Work out the finished part from the listing and answer in its coordinate system (mm). A direction names the side the tool comes from. Round coordinates to 2 decimals unless told otherwise and drop trailing zeros. Order: outer loops, then holes, each group sorted by start corner. A loop starts at its lowest first (then second) coordinate and runs counter-clockwise, first axis right, second up. Notation, with made-up numbers: (42.5, -9.75) - (75.5, -9.75) arc R17 ccw to (75.5, 22.25) - close; hole circle Ø7 at (3, -39). An arc over 180 degrees is marked (long way). Answer in a Markdown table with one row per item.
Autodesk Inventor part; units mm, degrees
ref_plane "YZ Plane" through (0, 0, 0) normal (1, 0, 0) x (0, 1, 0)
ref_plane "XZ Plane" through (0, 0, 0) normal (0, 1, 0) x (-1, 0, 0)
ref_plane "XY Plane" through (0, 0, 0) normal (0, 0, 1) x (1, 0, 0)
sketch "Sketch1" plane through (0, 0, 0) normal (0, 1, 0) x (-1, 0, 0)
  line L0 (0, 0) -> (-34, 0)
  line L1 (-34, 0) -> (-34, 34)
  line L2 (-34, 34) -> (0, 34)
  line L3 (0, 34) -> (0, 0)
  dimension "d0" = 34
  dimension "d1" = 34
extrude "Extrusion1" add sketch "Sketch1" along normal blind 33
sketch "Sketch2" plane through (0, 33, 0) normal (0, 1, 0) x (1, 0, 0)
  line L0 (0, -34) -> (34, -34)
  line L1 (34, -34) -> (34, 0)
  line L2 (34, 0) -> (0, 0)
  line L3 (0, 0) -> (0, -34)
  line L4 (2, -2) -> (32, -2)
  line L5 (32, -2) -> (32, -32)
  line L6 (32, -32) -> (2, -32)
  line L7 (2, -32) -> (2, -2)
  dimension "d4" = 2
extrude "Extrusion2" cut sketch "Sketch2" against normal blind 36 contours L4 L5 L6 L7
sketch "Sketch3" plane through (34, 0, 34) normal (1, 0, 0) x (0, 0, -1)
  line L0 (0, 0) -> (34, 0)
  line L1 (0, 33) -> (34, 33)
  line L2 (2, 33) -> (32, 33)
  line L3 (34, 0) -> (34, 38)
  line L4 (34, 0) -> (29, 0)
  line L5 (0, 0) -> (34, 0)
  line L6 (29, 0) -> (29, 4)
  line L7 (34, 0) -> (34, 33)
  line L8 (0, 0) -> (0, 33)
  line L9 (32, 0) -> (2, 0)
  line L10 (32, 33) -> (32, 0)
  line L11 (2, 33) -> (2, 0)
  dimension "d7" = 5
  dimension "d8" = 4
hole "Hole1" at (34, 4, 5) direction (-1, 0, 0) diameter 4 depth 2
ref_plane "Work Plane1" through (17, 33, 32) normal (1, 0, 0) x (0, 0, -1)
mirror "Mirror1" about plane through (17, 33, 32) normal (1, 0, 0) of "Hole1"
sketch "Sketch6" plane through (0, 33, 0) normal (0, 1, 0) x (1, 0, 0)
  point P0 (0, 0)
sketch "Sketch7" plane through (0, 0, 0) normal (0, -1, 0) x (1, 0, 0)
  line L0 (34, 0) -> (0, 0)
  line L1 (0, 34) -> (34, 34)
  line L2 (34, 0) -> (0, 0)
  line L3 (0, 0) -> (0, 34)
  line L4 (0, 34) -> (34, 34)
  line L5 (34, 34) -> (34, 0)
extrude "Extrusion5" add sketch "Sketch7" against normal blind 2
equation "\"BendRadius\" = Thickness"
equation "\"BendReliefWidth\" = Thickness"
equation "\"BendReliefDepth\" = 0.5 * Thickness"
equation "\"CornerReliefSize\" = 4 * Thickness"
equation "\"MinimumRemnant\" = 2 * Thickness"
equation "\"TransitionRadius\" = BendRadius"
equation "\"JacobiRadiusSize\" = Thickness"
equation "\"GapSize\" = Thickness"
properties part number "waterBallonHolderv1"
1) Find section D-D, the plane z = 13. Give the vertices of the cut face in (x, y), then the cut area to 3 significant figures.
Filled in:
| item | result |
|---|---|
| outline | (0, 0) - (34, 0) - (34, 33) - (32, 33) - (32, 2) - (2, 2) - (2, 33) - (0, 33) - close |
| area | 192 mm^2 |
2) The mould has two halves that part along Z. Classify faces 3 (the face through (1, 2, 5)), 4 (the face through (17, 16, 0)), 5 (the face through (34, 16, 17)), 6 (the face through (17, 2, 17)): released by +Z, released by -Z, zero draft, split by the parting line, or undercut.
Filled in:
| item | result |
|---|---|
| face 3 | undercut |
| face 4 | released by -Z |
| face 5 | zero draft |
| face 6 | undercut |
3) Find section B-B, the plane x = 26. Give the vertices of the cut face in (y, z).
Filled in:
| item | result |
|---|---|
| outline | (0, 0) - (33, 0) - (33, 2) - (2, 2) - (2, 32) - (33, 32) - (33, 34) - (0, 34) - close |
4) Each of these flat-tipped pins is pushed along its axis until it touches: pin 1 (8 mm diameter, centred on x = 7, z = 16, fed in from +Y); pin 2 (3 mm diameter, centred on y = 4, z = 5, fed in from -X). Where does it stop, or does it pass through?
Filled in:
| item | result |
|---|---|
| pin 1 | stops at y = 2 |
| pin 2 | passes through |
5) Find the intervals of material crossed by probe 1 along X at (y, z) = (20.5, 19); probe 2 along Y at (x, z) = (32.6, 5); probe 3 along Z at (x, y) = (1.45, 4), in increasing order. Write a range as from..to.
Filled in:
| item | result |
|---|---|
| probe 1 | x = 0..2, 32..34 |
| probe 2 | y = 0..2, 6..33 |
| probe 3 | z = 0..3, 7..34 |
6) Find section C-C, the plane y = 4. Give the vertices of the cut face in (x, z), then the cut area to 3 significant figures.
Filled in:
| item | result |
|---|---|
| outline | (0, 0) - (34, 0) - (34, 3) - (32, 3) - (32, 2) - (2, 2) - (2, 3) - (0, 3) - close; (0, 7) - (2, 7) - (2, 32) - (32, 32) - (32, 7) - (34, 7) - (34, 34) - (0, 34) - close |
| area | 240 mm^2 |
7) Find section A-A, the plane y = 27.5. Give the vertices of the cut face in (x, z).
Filled in:
| item | result |
|---|---|
| outline | (0, 0) - (34, 0) - (34, 34) - (0, 34) - close; hole (2, 2) - (32, 2) - (32, 32) - (2, 32) - close |
8) Which of the six approach directions +Z, -Z, +X, -X, +Y, -Y give full straight-line access (tool end or side, diameter ignored) to faces 1 (the face through (32.2, 33, 17.1)), 2 (the face through (17, 18, 2))?
Filled in:
| item | result |
|---|---|
| face 1 | +Z, -Z, +X, -X, +Y |
| face 2 | +Y |
